The model under review builds one solid part; all positions refer to its coordinate system, in mm. Face numbers are marked on the shaded views. A direction names the side the tool comes from. Give positions to 0.01 mm unless a question says otherwise; leave off trailing zeros. Order: outer loops, then holes, each group sorted by start corner. A loop starts at its lowest first (then second) coordinate and runs counter-clockwise, first axis right, second up. Notation, with made-up numbers: (68, -22.75) - (114, -22.75) arc R29 cw to (114, 4.25) - close; hole circle Ø7 at (-5, 74). An arc over 180 degrees is marked (long way). Use CSV: the item, a comma, the result in double quotes. Start each with the question number.
```python
from build123d import *

# Parameters (mm, degrees)
BOSS_EXTRUDE1_DEPTH      = 12.5
BOSS_EXTRUDE1_DEPTH_BACK = 12.5
SKETCH3_R                = 1.55
SKETCH3_R_2              = 1.7
CUT_EXTRUDE1_DEPTH       = 7.5
SKETCH4_W                = 22.85
SKETCH4_H                = 17.75
CUT_EXTRUDE2_DEPTH       = 5.75
SKETCH5_R                = 2
CUT_EXTRUDE3_DEPTH       = 5.75
SKETCH6_R                = 3.325
CUT_EXTRUDE4_DEPTH       = 3
SKETCH7_R                = 4.825
CUT_EXTRUDE5_DEPTH       = 3
SKETCH9_R                = 1.1
SKETCH9_W                = 8.2
SKETCH9_H                = 2.4
CUT_EXTRUDE6_DEPTH       = 8.2
SKETCH10_R               = 2
CUT_EXTRUDE7_DEPTH       = 8.2
SKETCH11_R               = 1
SKETCH11_W               = 8.2
SKETCH11_H               = 2
BOSS_EXTRUDE2_DEPTH      = 8
CUT_EXTRUDE8_DEPTH       = 23
CUT_EXTRUDE8_DEPTH_BACK  = 24
SKETCH13_R               = 2


with BuildPart() as part:
    # Sketch1 → Boss-Extrude1 (new, two sides: drawn at the far end of the back side and taken through both)
    with BuildSketch(Plane(origin=(0, 0, 0), x_dir=(1, 0, 0), z_dir=(0, 1, 0)).offset(-BOSS_EXTRUDE1_DEPTH_BACK)):
        with BuildLine():
            Line((7.5, -20), (-7.5, -20))
            ThreePointArc((-7.5, -20), (-27.5, 0), (-7.5, 20))
            Line((-7.5, 20), (7.5, 20))
            ThreePointArc((7.5, 20), (27.5, 0), (7.5, -20))
        make_face()
        with BuildLine():
            Line((-13.067764363, 15), (13.067764363, 15))
            ThreePointArc((13.067764363, 15), (23.297278294, 2.538897101), (17.487492178, -12.5))
            Line((17.487492178, -12.5), (-17.487492178, -12.5))
            ThreePointArc((-17.487492178, -12.5), (-23.297278294, 2.538897101), (-13.067764363, 15))
        make_face(mode=Mode.SUBTRACT)
    extrude(amount=BOSS_EXTRUDE1_DEPTH + BOSS_EXTRUDE1_DEPTH_BACK)

    # Sketch3 → Cut-Extrude1 (cut)
    with BuildSketch(Plane.XY.offset(20)):
        with Locations((-7.1, 0)):
            Circle(SKETCH3_R)
        with Locations((-2.9, 0)):
            Circle(SKETCH3_R)
        with Locations((1.3, 0)):
            Circle(SKETCH3_R)
        with Locations((6.95, 0)):
            Circle(SKETCH3_R_2)
    extrude(amount=-CUT_EXTRUDE1_DEPTH, mode=Mode.SUBTRACT)

    # Sketch4 → Cut-Extrude2 (cut)
    with BuildSketch(Plane(origin=(0, 0, 12.5), x_dir=(-1, 0, 0), z_dir=(0, 0, -1))):
        Rectangle(SKETCH4_W, SKETCH4_H)
    extrude(amount=-CUT_EXTRUDE2_DEPTH, mode=Mode.SUBTRACT)

    # Sketch5 → Cut-Extrude3 (cut)
    with BuildSketch(Plane(origin=(0, 0, 12.5), x_dir=(-1, 0, 0), z_dir=(0, 0, -1))):
        with Locations((14.925, 0)):
            Circle(SKETCH5_R)
        with Locations((-14.925, 0)):
            Circle(SKETCH5_R)
    extrude(amount=-CUT_EXTRUDE3_DEPTH, mode=Mode.SUBTRACT)

    # Sketch6 → Cut-Extrude4 (cut)
    with BuildSketch(Plane.XY.offset(20)):
        with Locations((-14.925, 0)):
            Circle(SKETCH6_R)
        with Locations((14.925, 0)):
            Circle(SKETCH6_R)
    extrude(amount=-CUT_EXTRUDE4_DEPTH, mode=Mode.SUBTRACT)

    # Sketch7 → Cut-Extrude5 (cut)
    with BuildSketch(Plane(origin=(0, 0, 12.5), x_dir=(-1, 0, 0), z_dir=(0, 0, -1))):
        with Locations((14.925, 0)):
            Circle(SKETCH7_R)
        with Locations((-14.925, 0)):
            Circle(SKETCH7_R)
    extrude(amount=CUT_EXTRUDE5_DEPTH, mode=Mode.SUBTRACT)

    # Sketch9 → Cut-Extrude6 (cut)
    with BuildSketch(Plane.XZ.offset(12.5)):
        with Locations(Location((22.466629547, 10, 0), (0, 0, 270))):
            Circle(SKETCH9_R)
        with Locations(Location((22.466629547, -10, 0), (0, 0, 270))):
            Circle(SKETCH9_R)
        with Locations((0, -16.2)):
            Rectangle(SKETCH9_W, SKETCH9_H)
        with BuildLine():
            Line((-7.5, 14.9), (-7.5, 17.1))
            ThreePointArc((-7.5, 17.1), (-24.6, 0), (-7.5, -17.1))
            Line((-7.5, -17.1), (-7.5, -14.9))
            ThreePointArc((-7.5, -14.9), (-22.4, 0), (-7.5, 14.9))
        make_face()
    extrude(amount=-CUT_EXTRUDE6_DEPTH, mode=Mode.SUBTRACT)

    # Sketch10 → Cut-Extrude7 (cut)
    with BuildSketch(Plane.XY.offset(-17.4)):
        with Locations((0, -8.4)):
            Circle(SKETCH10_R)
    extrude(amount=-CUT_EXTRUDE7_DEPTH, mode=Mode.SUBTRACT)

    # Sketch11 → Boss-Extrude2 (add)
    with BuildSketch(Plane(origin=(0, 12.5, 0), x_dir=(1, 0, 0), z_dir=(0, 1, 0))):
        with Locations(Location((22.466629547, -10, 0), (0, 0, 270))):
            Circle(SKETCH11_R)
        with Locations(Location((22.466629547, 10, 0), (0, 0, 270))):
            Circle(SKETCH11_R)
        with BuildLine():
            Line((-8.5, -14.966629547), (-8.5, -16.970562748))
            ThreePointArc((-8.5, -16.970562748), (-14.464941324, -15.50772686), (-19.52081528, -12.02081528))
            Line((-19.52081528, -12.02081528), (-18.106601718, -10.606601718))
            ThreePointArc((-18.106601718, -10.606601718), (-13.699254917, -13.659035049), (-8.5, -14.966629547))
        make_face()
        with BuildLine():
            Line((-18.106601718, 10.606601718), (-19.52081528, 12.02081528))
            ThreePointArc((-19.52081528, 12.02081528), (-14.464941324, 15.50772686), (-8.5, 16.970562748))
            Line((-8.5, 16.970562748), (-8.5, 14.966629547))
            ThreePointArc((-8.5, 14.966629547), (-13.699254917, 13.659035049), (-18.106601718, 10.606601718))
        make_face()
        with Locations((0, 16)):
            Rectangle(SKETCH11_W, SKETCH11_H)
        with Locations((0, -16.25)):
            Rectangle(SKETCH11_W, SKETCH11_H)
    extrude(amount=BOSS_EXTRUDE2_DEPTH)

    # Sketch13 → Cut-Extrude8 (cut, two sides: drawn at the far end of the back side and taken through both)
    with BuildSketch(Plane.XY.offset(-CUT_EXTRUDE8_DEPTH_BACK)):
        with Locations(Location((0, 16.5, 0), (0, 0, 180))):
            Circle(SKETCH13_R)
    extrude(amount=CUT_EXTRUDE8_DEPTH + CUT_EXTRUDE8_DEPTH_BACK, mode=Mode.SUBTRACT)


solid = part.part
```
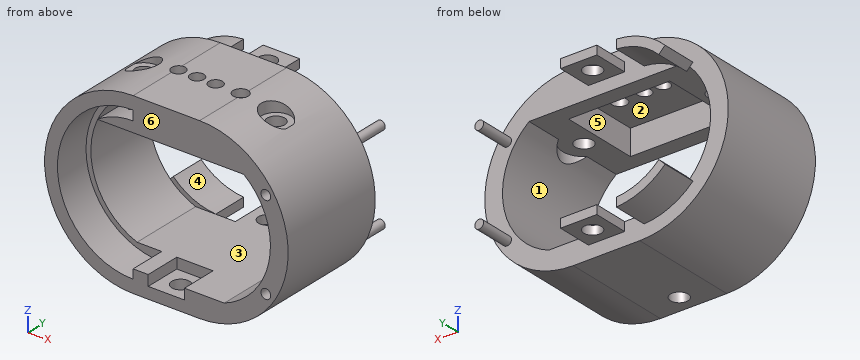
1. Consider section D-D (z = -10). Give the boundary of the cut face in (x, y), and give its area (3 significant figures).
2. Consider section A-A (x = -2.9). Give the boundary of the cut face in (y, z) (3 decimals).
3. Mouldability with a two-part tool opening along Y and no side actions: class the marked faces 4, 5 and 6 as pulls with the +Y half, pulls with the -Y half, needs draft (parallel to the pull), parting line crosses it, or undercut.
4. Consider section B-B (z = 1.5). Give the boundary of the cut face in (x, y), and give its area (3 significant figures).
5. Clearance check with flat-ended pins moving along their axes: pin 1 (5 mm diameter, centred on x = 0, y = 16.5, fed in from +Z); pin 2 (2 mm diameter, centred on y = 1.5, z = -9, fed in from +X); pin 3 (5 mm diameter, centred on x = -18, y = 14, fed in from +Z). State where each tip first meets the part, or that it passes through.
6. Consider section C-C (x = 9.5). Give the boundary of the cut face in (y, z) (3 decimals).
7. To check wall thickness, follow L1, parallel to Z at x = -8, y = 2.5; L2, parallel to X at y = 0, z = 18 (3 decimals); L3, parallel to Z at x = 1, y = 0.5. State the ranges of each line that lie inside material, in increasing order. Write a range as [from, to].
8. Tool access review of the marked faces 1, 2 and 3: name each direction out of +Z, -Z, +X, -X, +Y, -Y from which nothing blocks a thin tool from reaching the whole face with its end or side.
Answers follow:
1,outline,"(-24.82, -12.5) - (-21.37, -12.5) - (-21.37, -4.3) - (-19.99, -4.3) - (-19.99, 12.5) - (-24.82, 12.5) - close; (19.99, -12.5) - (21.37, -12.5) - (21.37, -4.3) - (23.57, -4.3) - (23.57, -12.5) - (24.82, -12.5) - (24.82, 12.5) - (23.47, 12.5) - (23.47, 20.5) - (21.47, 20.5) - (21.47, 12.5) - (19.99, 12.5) - close"
1,area,"228 mm^2"
2,outline,"(-12.5, -20) - (12.5, -20) - (12.5, -17) - (20.5, -17) - (20.5, -15) - (-4.3, -15) - (-4.3, -17.4) - (-12.5, -17.4) - close; (-12.5, 12.5) - (-8.875, 12.5) - (-8.875, 18.25) - (-1.55, 18.25) - (-1.55, 20) - (-12.5, 20) - close; (1.55, 18.25) - (8.875, 18.25) - (8.875, 12.5) - (12.5, 12.5) - (12.5, 15.25) - (20.5, 15.25) - (20.5, 17.25) - (12.5, 17.25) - (12.5, 20) - (1.55, 20) - close"
3,face 4,"needs draft"
3,face 5,"undercut"
3,face 6,"pulls with the -Y half"
4,outline,"(-27.44, -12.5) - (-24.53, -12.5) - (-24.53, -4.3) - (-23.43, -4.3) - (-23.43, 12.5) - (-27.44, 12.5) - close; (23.43, -12.5) - (27.44, -12.5) - (27.44, 12.5) - (23.43, 12.5) - close"
4,area,"192 mm^2"
5,pin 1,"stops at z = 17.25"
5,pin 2,"stops at x = 25.83"
5,pin 3,"stops at z = 18.1"
6,outline,"(-12.5, -19.9) - (12.5, -19.9) - (12.5, -15) - (-12.5, -15) - close; (-12.5, 12.5) - (-8.875, 12.5) - (-8.875, 18.25) - (8.875, 18.25) - (8.875, 12.5) - (12.5, 12.5) - (12.5, 19.9) - (-12.5, 19.9) - close"
7,L1,"z = [-19.99, -15], [18.25, 19.99]"
7,L2,"x = [-11.6, -11.425], [11.425, 11.6]"
7,L3,"z = [-20, -15]"
8,face 1,"+Y, -Y"
8,face 2,"none"
8,face 3,"-Y"
